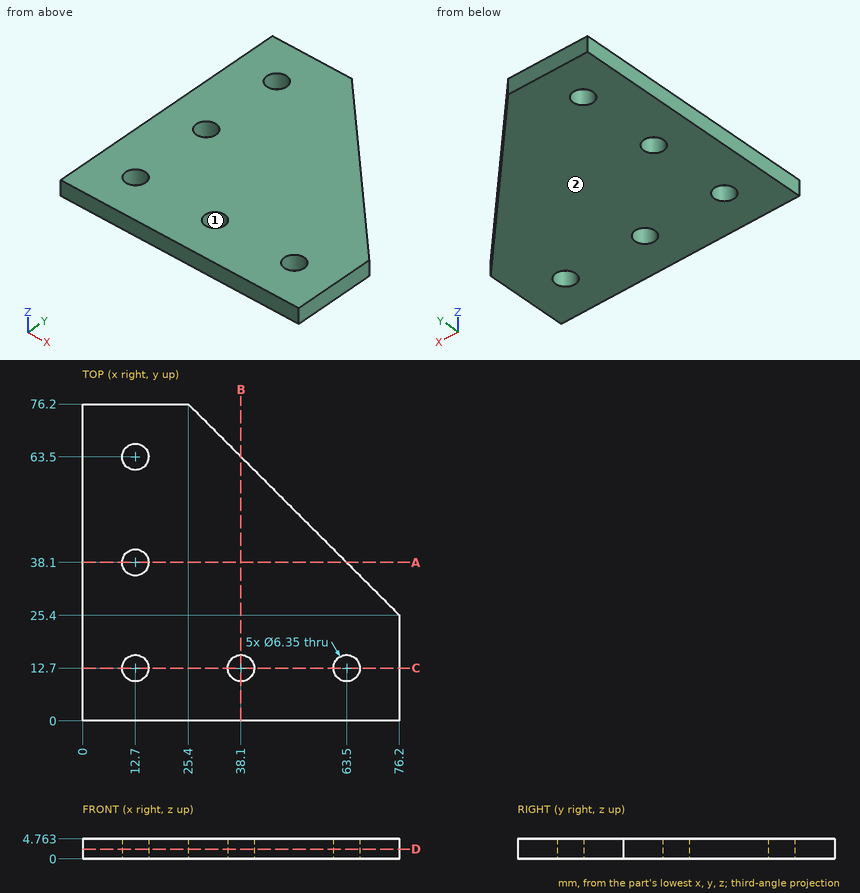
Answer from the drawing. Dimensions are ordinates in mm from the lowest x, y and z of the part. Coordinates: 2 decimals unless noted, no trailing zeros. Write each loop counter-clockwise with the first axis right and the second up, starting at its lowest first coordinate (ties: lowest second). Pieces come first, ordered by that corner, then holes. Notation, with made-up numbers: (6.5, 67.5) -> (25.5, 67.5) arc R13 ccw to (25.5, 87.5) -> close; hole circle Ø11 at (85.5, 79.25). An arc over 180 degrees is marked (long way). One line per question, with ' | ' between items.
1. Given pin 1 Ø4 at (x, y) = (12.7, 38.1) entering from -Z, flat-ended and moving along its own axis, determine where the tip first touches the part or whether it passes through.
Verdict:
pin 1: passes through
2. For a pull along Y with two mould halves and no side action, classify the marked faces 1 and 2 as released by +Y, released by -Y, zero draft, split by the parting line, or undercut.
Verdict:
face 1: undercut | face 2: zero draft
3. Section C-C (y = 12.7) is taken. Determine the outline of the cut face in (x, z) (1 decimal), and give its area (3 significant figures).
Verdict:
outline: (0, 0) -> (9.5, 0) -> (9.5, 4.8) -> (0, 4.8) -> close; (15.9, 0) -> (34.9, 0) -> (34.9, 4.8) -> (15.9, 4.8) -> close; (41.3, 0) -> (60.3, 0) -> (60.3, 4.8) -> (41.3, 4.8) -> close; (66.7, 0) -> (76.2, 0) -> (76.2, 4.8) -> (66.7, 4.8) -> close | area: 272 mm^2
4. Straight lines are drawn through the part: line 1 (X direction, y = 12.7, z = 1.5) (1 decimal); line 2 (X direction, y = 41, z = 3.45) (1 decimal). For each, find the intervals that lie inside material, in ascending order.
Verdict:
line 1: x = 0 to 9.5, 15.9 to 34.9, 41.3 to 60.3, 66.7 to 76.2 | line 2: x = 0 to 11.4, 14 to 60.6
5. Section D-D (z = 2.35) is taken. State how many separate pieces and enclosed holes the cut face has, and give its area (3 significant figures).
Verdict:
separate pieces: 1 | enclosed holes: 5 | area: 4,360 mm^2
6. Section A-A (y = 38.1) is taken. Determine the outline of the cut face in (x, z) (1 decimal), and give its area (3 significant figures).
Verdict:
outline: (0, 0) -> (9.5, 0) -> (9.5, 4.8) -> (0, 4.8) -> close; (15.9, 0) -> (63.5, 0) -> (63.5, 4.8) -> (15.9, 4.8) -> close | area: 272 mm^2
